Can you work these out from the model? Positions are in its coordinate system, mm. A direction names the side the tool comes from. Coordinates: 2 decimals unless noted, no trailing zeros. Order: outer loops, then holes, each group sorted by start corner. A loop starts at its lowest first (then second) coordinate and runs counter-clockwise, first axis right, second up. Notation, with made-up numbers: M -30.75,-37.75 L 27.25,-37.75 A18 ccw 27.25,-3.75 Z; hole C -7.75,-19 d9. An arc over 180 degrees is marked long. Answer as a JSON object with one key per item and string values.
from build123d import *

# Parameters (mm, degrees)
PAD_DEPTH = 10


with BuildPart() as part:
    # Sketch → Pad (new body)
    with BuildSketch(Plane.XY):
        Polygon((-1e-05, 59.5), (5.99999, 59.5), (29.389263, 40.45085), (34.973223, 48.136511), (39.643333, 44.369541), (47.552826, 15.45085), (56.587863, 18.386511), (58.151892, 12.593946), (47.552826, -15.45085), (56.587863, -18.386511), (54.448404, -23.992108), (29.389263, -40.45085), (34.973223, -48.136511), (29.947477, -51.413992), (0, -50), (0, -59.5), (-6, -59.5), (-29.389263, -40.45085), (-34.973223, -48.136511), (-39.643333, -44.369541), (-47.552826, -15.45085), (-56.587863, -18.386511), (-58.151892, -12.593946), (-47.552826, 15.45085), (-56.587863, 18.386511), (-54.448404, 23.992108), (-29.389263, 40.45085), (-34.973223, 48.136511), (-29.947477, 51.413992), (-1e-05, 50), align=None)
        with BuildLine():
            ThreePointArc((28.01339, 7.5), (-29, 0), (28.01339, -7.5))
            Line((35.721142, -7.5), (28.01339, -7.5))
            Line((35.721142, 7.5), (35.721142, -7.5))
            Line((28.01339, 7.5), (35.721142, 7.5))
        make_face(mode=Mode.SUBTRACT)
    extrude(amount=PAD_DEPTH)


solid = part.part
Item 1: Please list where these lines run through material, in increasing order: line 1 (Y direction, x = 32.5, z = 7.75); line 2 (X direction, y = 0, z = 4); line 3 (X direction, y = 15, z = 3).
Answers follow:
{"line 1": "y = -49.75 to -44.73, -38.41 to -7.5, 7.5 to 44.73", "line 2": "x = -53.39 to -29, 35.72 to 53.39", "line 3": "x = -47.72 to -24.82, 24.82 to 57.5"}
Item 2: I'm going to push flat-ended pins straight in: pin 1 (6 mm diameter, centred on x = -5.5, z = 2, fed in from +Y); pin 2 (2.5 mm diameter, centred on x = 31, z = 2.5, fed in from -Y); pin 3 (1.5 mm diameter, centred on y = 0.5, z = 3.5, fed in from -X). Where does each tip first touch, or does it pass through?
Answers follow:
{"pin 1": "stops at y = 50.4", "pin 2": "stops at y = -51.41", "pin 3": "stops at x = -53.49"}
Item 3: I want a section at B-B, the plane y = 0. Write out the boundary of the cut face in (x, z).
Answers follow:
{"outline": "M -53.39,0 L -29,0 L -29,10 L -53.39,10 Z; M 35.72,0 L 53.39,0 L 53.39,10 L 35.72,10 Z"}
Item 4: If we mould it in two halves opening along Y, with no side actions, what happens to faces 5 (the flat face through (32.14, -44.24, 4.93)), 6 (the flat face through (15.183, -50.717, 4.93)), 7 (the flat face through (0, -55, 5))? For each: pulls with the +Y half, pulls with the -Y half, needs draft (parallel to the pull), parting line crosses it, or undercut.
Answers follow:
{"face 5": "undercut", "face 6": "pulls with the -Y half", "face 7": "needs draft"}
Item 5: Which directions (+Z, -Z, +X, -X, +Y, -Y) give clear straight access to the entire face, cutting with the end or side of a thin tool? Please do faces 1 (the flat face through (52.01, -16.9, 4.93)), 2 (the flat face through (-32.14, 44.24, 4.93)), 3 (the flat face through (17.53, 50.11, 4.93)), 4 (the flat face through (32, 7.5, 5)).
Answers follow:
{"face 1": "+Z, -Z, +X", "face 2": "+Z, -Z, -X", "face 3": "+Z, -Z, +Y", "face 4": "+Z, -Z"}
Item 6: I want a section at A-A, the plane x = 21.5. Write out the boundary of the cut face in (y, z).
Answers follow:
{"outline": "M -51.02,0 L -19.46,0 L -19.46,10 L -51.02,10 Z; M 19.46,0 L 46.88,0 L 46.88,10 L 19.46,10 Z"}
Item 7: I want a section at D-D, the plane y = -17. Write out the boundary of the cut face in (x, z).
Answers follow:
{"outline": "M -56.96,0 L -52.32,0 L -52.32,10 L -56.96,10 Z; M -47.13,0 L -23.49,0 L -23.49,10 L -47.13,10 Z; M 23.49,0 L 52.32,0 L 52.32,10 L 23.49,10 Z"}
